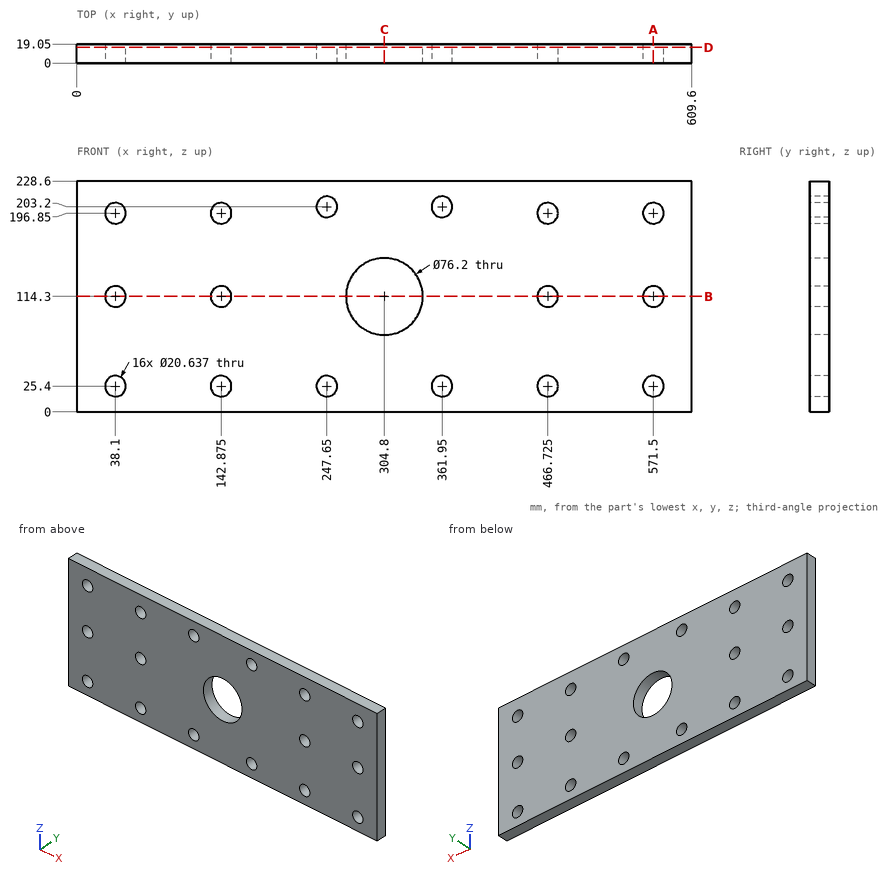
Study the drawing (mm; zero at the part's minimum x, y, z) and answer. Give positions to 0.01 mm unless a question says otherwise; leave off trailing zeros. Loops run counter-clockwise (first coordinate to the right, second up) from the corner with the lowest first, then second, coordinate; pieces in that order, holes last. Notation, with made-up numbers: M -26,42.25 L 15,42.25 A22 ccw 15,67.25 Z; hole C -5.5,-14 d11. An arc over 180 degrees is marked long. One line per item, written item: value.
1. Find the intervals of material crossed by probe 1 along Z at (x, y) = (571.5, 9); probe 2 along X at (y, z) = (3.5, 191) (1 decimal); probe 3 along X at (y, z) = (4.25, 118), in increasing order.
Found:
probe 1: 0 to 15.08, 35.72 to 103.98, 124.62 to 186.53, 207.17 to 228.6
probe 2: 0 to 29.6, 46.6 to 134.4, 151.4 to 458.2, 475.2 to 563, 580 to 609.6
probe 3: 0 to 28.47, 47.73 to 133.24, 152.51 to 266.88, 342.72 to 457.09, 476.36 to 561.87, 581.13 to 609.6
2. Section D-D on y = 15.75 is taken. State how many separate pieces and enclosed holes the cut face has, plus the area to 3 significant figures.
Found:
separate pieces: 1
enclosed holes: 17
area: 129,000 mm^2
3. Section B-B on z = 114.3 is taken. Determine the outline of the cut face in (x, y).
Found:
outline: M 0,0 L 27.78,0 L 27.78,19.05 L 0,19.05 Z; M 48.42,0 L 132.56,0 L 132.56,19.05 L 48.42,19.05 Z; M 153.19,0 L 266.7,0 L 266.7,19.05 L 153.19,19.05 Z; M 342.9,0 L 456.41,0 L 456.41,19.05 L 342.9,19.05 Z; M 477.04,0 L 561.18,0 L 561.18,19.05 L 477.04,19.05 Z; M 581.82,0 L 609.6,0 L 609.6,19.05 L 581.82,19.05 Z
4. This flat-tipped pin is pushed along its axis until it touches: P1, Ø23.5, axis at x = 571.5, z = 114.3, coming from the +Y side. Where does it stop, or does it pass through?
Found:
P1: y = 19.05
5. Section C-C on x = 304.8 is taken. Determine the outline of the cut face in (y, z).
Found:
outline: M 0,0 L 19.05,0 L 19.05,76.2 L 0,76.2 Z; M 0,152.4 L 19.05,152.4 L 19.05,228.6 L 0,228.6 Z
6. Section A-A on x = 571.5 is taken. Determine the outline of the cut face in (y, z).
Found:
outline: M 0,0 L 19.05,0 L 19.05,15.08 L 0,15.08 Z; M 0,35.72 L 19.05,35.72 L 19.05,103.98 L 0,103.98 Z; M 0,124.62 L 19.05,124.62 L 19.05,186.53 L 0,186.53 Z; M 0,207.17 L 19.05,207.17 L 19.05,228.6 L 0,228.6 Z
